Check sheet for the modelled part. Datum: model origin and axes. Units: mm. Face numbers are marked on the shaded views. A direction names the side the tool comes from. Round coordinates to 2 decimals unless told otherwise and drop trailing zeros. Loops run counter-clockwise (first coordinate to the right, second up) from the corner with the lowest first, then second, coordinate; pieces in that order, holes last. Notation, with made-up numbers: (-38.75, 43.25) -> (-18.75, 43.25) arc R18 ccw to (-18.75, 76.25) -> close; hole circle Ø3 at (-8, 23). An arc over 180 degrees is marked (long way). Use one line per item in the form item = value. Start each with the question number.
(1) Draft check along X on the marked faces 1 and 2. Enter one of: released by +X, released by -X, zero draft, split by the parting line, or undercut.
(2) Sectioned sample at B-B (x = 0). Record the cut outline in (y, z), and give its area (3 significant figures).
(3) Material ranges on probe 1 along X at (y, z) = (53.75, 10.9); probe 2 along Y at (x, z) = (-17.65, 0.2); probe 3 along X at (y, z) = (48.5, 0.7), recorded low to high. Write a range as [from, to].
(4) Sectioned sample at A-A (y = 31). Record the cut outline in (x, z), and give its area (3 significant figures).
(5) Sectioned sample at C-C (y = -53.75). Record the cut outline in (x, z), and give its area (3 significant figures).
(6) Go/stop test with flat-tipped pins: pin 1 (4 mm diameter, centred on x = 17.65, y = 13.5, fed in from +Z); pin 2 (6 mm diameter, centred on x = 76.5, y = 0, fed in from -Z); pin 3 (4 mm diameter, centred on y = -27.5, z = 3, fed in from -X). Record where each tip stops, or that it passes through.
(7) Sectioned sample at D-D (y = 59). Record the cut outline in (x, z), and give its area (3 significant figures).
(8) Set-up check for the marked faces 3, 4 and 5: record each of +Z, -Z, +X, -X, +Y, -Y from which the full face is reachable in a straight line by a thin tool's end or side.
Autodesk Fusion 360 part; units mm, degrees
sketch "extrusion" plane through (0, 0, 0) normal (0, 1, 0) x (1, 0, 0)
  line L0 (-82.5, -8) -> (-62.5, -8)
  line L1 (-62.5, -8) -> (-62.5, 0)
  line L2 (-62.5, 0) -> (62.5, 0)
  line L3 (62.5, 0) -> (62.5, -8)
  line L4 (62.5, -8) -> (82.5, -8)
  line L5 (-60.5, -12) -> (-60.5, -2)
  line L6 (-60.5, -2) -> (60.5, -2)
  line L7 (60.5, -2) -> (60.5, -12)
  line L8 (-82.5, -12) -> (-60.5, -12)
  line L9 (60.5, -12) -> (82.5, -12)
  line L10 (-82.5, -8) -> (-82.5, -12)
  line L11 (82.5, -8) -> (82.5, -12)
  dimension "d1" = 125
  dimension "d2" = 8
  dimension "d3" = 20
  dimension "d4" = 8
  dimension "d5" = 20
extrude "Extrude1" add sketch "extrusion" along normal mid plane 140
sketch "top holes" plane through (0, 0, 12) normal (0, 0, 1) x (-1, 0, 0)
  circle A0 centre (71.5, -53.75) radius 3
  line L0 (82.5, -70) -> (60.5, -70)
  dimension "d11" = 6
  dimension "d12" = 16.25
extrude "Extrude2" cut sketch "top holes" against normal blind 4
mirror "Mirror1" about plane through (0, 0, 0) normal (1, 0, 0) of "Extrude2"
mirror "Mirror2" about plane through (0, 0, 0) normal (0, 1, 0) of "Extrude2", "Mirror1"
sketch "square undent" plane through (0, 0, 2) normal (0, 0, 1) x (-1, 0, 0)
  line L0 (22.5, -53.5) -> (-22.5, -53.5)
  line L1 (-22.5, -53.5) -> (-22.5, -8.5)
  line L2 (-22.5, -8.5) -> (22.5, -8.5)
  line L3 (22.5, -8.5) -> (22.5, -53.5)
  line L4 (60.5, -70) -> (-60.5, -70)
  dimension "d17" = 45
  dimension "d18" = 45
  dimension "d19" = 16.5
extrude "Extrude3" cut sketch "square undent" against normal blind 1
sketch "square holes" plane through (0, 0, 1) normal (0, 0, 1) x (-1, 0, 0)
  circle A0 centre (17.65, -48.5) radius 1.75
  line L0 (22.5, -53.5) -> (-22.5, -53.5)
  line L1 (22.5, -8.5) -> (22.5, -53.5)
  line L2 (-22.5, -8.5) -> (22.5, -53.5) construction
  circle A1 centre (0, -31) radius 16
  arc A2 (4.2359, -30.0006) -> (0, -15) centre (-16.1329, -27.654) ccw
  arc A3 (6.0614, -30.6697) -> (7.9315, -17.1043) centre (-7.0111, -21.9559) ccw
  arc A4 (4.2359, -30.0006) -> (6.0614, -30.6697) centre (5.2293, -30.115) ccw
  dimension "d22" = 3.5
  dimension "d23" = 5
  dimension "d24" = 4.85
  dimension "d25" = 32
  dimension "d26" = 1
extrude "Extrude4" cut sketch "square holes" against normal blind 1 contours A0
ref_plane "WorkPlane1" through (0, 31, 1.5) normal (0, -1, 0) x (-1, 0, 0)
mirror "Mirror3" about plane through (0, 31, 1.5) normal (0, -1, 0) of "Extrude4"
mirror "Mirror4" about plane through (0, 0, 0) normal (1, 0, 0) of "Extrude4", "Mirror3"
extrude "Extrude5" cut sketch "square holes" against normal blind 1 contours A1 A2 A3 A4 picked at (-1.7065, -26.7053)
pattern_circular "C-Pattern1" count 5 over 360 about axis through (0, 31, 1) along (0, 0, -1) of "Extrude5"
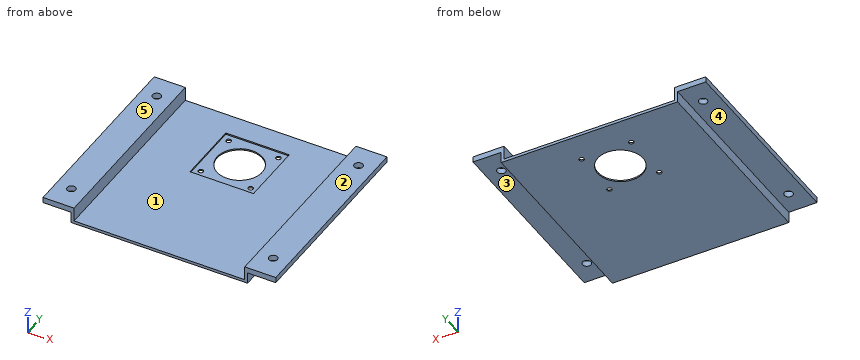
Checks:
q1.face_1 = undercut
q1.face_2 = zero draft
q2.outline = (-70, 0) -> (15, 0) -> (15, 1) -> (8.5, 1) -> (8.5, 2) -> (-70, 2) -> close; (47, 0) -> (70, 0) -> (70, 2) -> (53.5, 2) -> (53.5, 1) -> (47, 1) -> close
q2.area = 203 mm2
q3.probe_1 = [-82.5, -74.5], [-68.5, -60.5], [60.5, 68.5], [74.5, 82.5]
q3.probe_2 = [-70, 11.75], [15.25, 46.75], [50.25, 70]
q3.probe_3 = [-62.5, -19.4], [-15.9, 15.9], [19.4, 62.5]
q4.outline = (-82.5, 8) -> (-62.5, 8) -> (-62.5, 0) -> (-16, 0) -> (-16, 1) -> (-22.5, 1) -> (-22.5, 2) -> (-60.5, 2) -> (-60.5, 12) -> (-82.5, 12) -> close; (16, 0) -> (62.5, 0) -> (62.5, 8) -> (82.5, 8) -> (82.5, 12) -> (60.5, 12) -> (60.5, 2) -> (22.5, 2) -> (22.5, 1) -> (16, 1) -> close
q4.area = 373 mm2
q5.outline = (-82.5, 8) -> (-74.5, 8) -> (-74.5, 12) -> (-82.5, 12) -> close; (-68.5, 8) -> (-62.5, 8) -> (-62.5, 0) -> (62.5, 0) -> (62.5, 8) -> (68.5, 8) -> (68.5, 12) -> (60.5, 12) -> (60.5, 2) -> (-60.5, 2) -> (-60.5, 12) -> (-68.5, 12) -> close; (74.5, 8) -> (82.5, 8) -> (82.5, 12) -> (74.5, 12) -> close
q5.area = 402 mm2
q6.pin_1 = 1
q6.pin_2 = 8
q6.pin_3 = -62.5
q7.outline = (-82.5, 8) -> (-62.5, 8) -> (-62.5, 0) -> (62.5, 0) -> (62.5, 8) -> (82.5, 8) -> (82.5, 12) -> (60.5, 12) -> (60.5, 2) -> (-60.5, 2) -> (-60.5, 12) -> (-82.5, 12) -> close
q7.area = 450 mm2
q8.face_3 = -Z, +X, +Y, -Y
q8.face_4 = -Z, -X, +Y, -Y
q8.face_5 = +Z, +X, -X, +Y, -Y
